```python
from build123d import *

# Parameters (mm, degrees)
BOSS_EXTRUDE2_DEPTH = 1000
CUT_EXTRUDE1_REACH  = 1002
SKETCH3_R           = 2
SKETCH3_R_2         = 1.999999992


with BuildPart() as part:
    # Sketch2 → Boss-Extrude2 (new body)
    with BuildSketch(Plane.XY):
        Polygon((0, 0), (0, 10), (0.7, 10), (0.7, 10.9), (2.2, 10.9), (2.2, 6.4), (4.9, 6.4), (9.142640687, 10.642640687), (9.142640687, 19.642640687), (4.9, 23.885281374), (2.2, 23.885281374), (2.2, 19.385281374), (0.7, 19.385281374), (0.7, 20.285281374), (0, 20.285281374), (0, 30.285281374), (10, 30.285281374), (10, 29.585281374), (10.9, 29.585281374), (10.9, 28.085281374), (6.4, 28.085281374), (6.4, 25.385281374), (10.642640687, 21.142640687), (19.642640687, 21.142640687), (23.885281374, 25.385281374), (23.885281374, 28.085281374), (19.385281374, 28.085281374), (19.385281374, 29.585281374), (20.285281374, 29.585281374), (20.285281374, 30.285281374), (30.285281374, 30.285281374), (30.285281374, 20.285281374), (29.585281374, 20.285281374), (29.585281374, 19.385281374), (28.085281374, 19.385281374), (28.085281374, 23.885281374), (25.385281374, 23.885281374), (21.142640687, 19.642640687), (21.142640687, 10.642640687), (25.385281374, 6.4), (28.085281374, 6.4), (28.085281374, 10.9), (29.585281374, 10.9), (29.585281374, 10), (30.285281374, 10), (30.285281374, 0), (20.285281374, 0), (20.285281374, 0.7), (19.385281374, 0.7), (19.385281374, 2.2), (23.885281374, 2.2), (23.885281374, 4.9), (19.642640687, 9.142640687), (10.642640687, 9.142640687), (6.4, 4.9), (6.4, 2.2), (10.9, 2.2), (10.9, 0.7), (10, 0.7), (10, 0), align=None)
    extrude(amount=-BOSS_EXTRUDE2_DEPTH)

    # Sketch3 → Cut-Extrude1 (cut, up to next)
    with BuildSketch(Plane.XY, mode=Mode.PRIVATE) as cut_extrude1_sk1:
        with Locations((3.200056686, 27.085348905)):
            Circle(SKETCH3_R)
    cut_extrude1_tool1 = extrude(cut_extrude1_sk1.sketch, amount=-CUT_EXTRUDE1_REACH, mode=Mode.PRIVATE) & part.part
    add(cut_extrude1_tool1.solids().sort_by_distance((3.200057, 27.085349, 0))[0], mode=Mode.SUBTRACT)
    # Sketch3 → Cut-Extrude1 (cut, up to next)
    with BuildSketch(Plane.XY, mode=Mode.PRIVATE) as cut_extrude1_sk2:
        with Locations((27.085224689, 27.085348905)):
            Circle(SKETCH3_R)
    cut_extrude1_tool2 = extrude(cut_extrude1_sk2.sketch, amount=-CUT_EXTRUDE1_REACH, mode=Mode.PRIVATE) & part.part
    add(cut_extrude1_tool2.solids().sort_by_distance((27.085225, 27.085349, 0))[0], mode=Mode.SUBTRACT)
    # Sketch3 → Cut-Extrude1 (cut, up to next)
    with BuildSketch(Plane.XY, mode=Mode.PRIVATE) as cut_extrude1_sk3:
        with Locations((27.085224689, 3.19993247)):
            Circle(SKETCH3_R)
    cut_extrude1_tool3 = extrude(cut_extrude1_sk3.sketch, amount=-CUT_EXTRUDE1_REACH, mode=Mode.PRIVATE) & part.part
    add(cut_extrude1_tool3.solids().sort_by_distance((27.085225, 3.199932, 0))[0], mode=Mode.SUBTRACT)
    # Sketch3 → Cut-Extrude1 (cut, up to next)
    with BuildSketch(Plane.XY, mode=Mode.PRIVATE) as cut_extrude1_sk4:
        with Locations((3.19993247, 3.200056686)):
            Circle(SKETCH3_R_2)
    cut_extrude1_tool4 = extrude(cut_extrude1_sk4.sketch, amount=-CUT_EXTRUDE1_REACH, mode=Mode.PRIVATE) & part.part
    add(cut_extrude1_tool4.solids().sort_by_distance((3.199932, 3.200057, 0))[0], mode=Mode.SUBTRACT)
    # Sketch3 → Cut-Extrude1 (cut, up to next)
    with BuildSketch(Plane.XY, mode=Mode.PRIVATE) as cut_extrude1_sk5:
        with BuildLine():
            Line((11.288922887, 17.865021836), (12.349577543, 16.804356148))
            ThreePointArc((12.349577543, 16.804356148), (11.892640687, 15.142640687), (12.349577543, 13.480925226))
            Line((12.349577543, 13.480925226), (11.288922887, 12.420259538))
            ThreePointArc((11.288922887, 12.420259538), (11.288928771, 11.288888688), (12.420299621, 11.288894572))
            Line((12.420299621, 11.288894572), (13.480954277, 12.34956026))
            ThreePointArc((13.480954277, 12.34956026), (15.142640687, 11.892640687), (16.804327097, 12.34956026))
            Line((16.804327097, 12.34956026), (17.864981753, 11.288894572))
            ThreePointArc((17.864981753, 11.288894572), (18.996352603, 11.288888688), (18.996358487, 12.420259538))
            Line((18.996358487, 12.420259538), (17.935703831, 13.480925226))
            ThreePointArc((17.935703831, 13.480925226), (18.392640687, 15.142640687), (17.935703831, 16.804356148))
            Line((17.935703831, 16.804356148), (18.996358487, 17.865021836))
            ThreePointArc((18.996358487, 17.865021836), (18.996352603, 18.996392686), (17.864981753, 18.996386802))
            Line((17.864981753, 18.996386802), (16.804327097, 17.935721114))
            ThreePointArc((16.804327097, 17.935721114), (15.142640687, 18.392640687), (13.480954277, 17.935721114))
            Line((13.480954277, 17.935721114), (12.420299621, 18.996386802))
            ThreePointArc((12.420299621, 18.996386802), (11.288928771, 18.996392686), (11.288922887, 17.865021836))
        make_face()
    cut_extrude1_tool5 = extrude(cut_extrude1_sk5.sketch, amount=-CUT_EXTRUDE1_REACH, mode=Mode.PRIVATE) & part.part
    add(cut_extrude1_tool5.solids().sort_by_distance((15.142641, 15.142641, 0))[0], mode=Mode.SUBTRACT)


solid = part.part
```
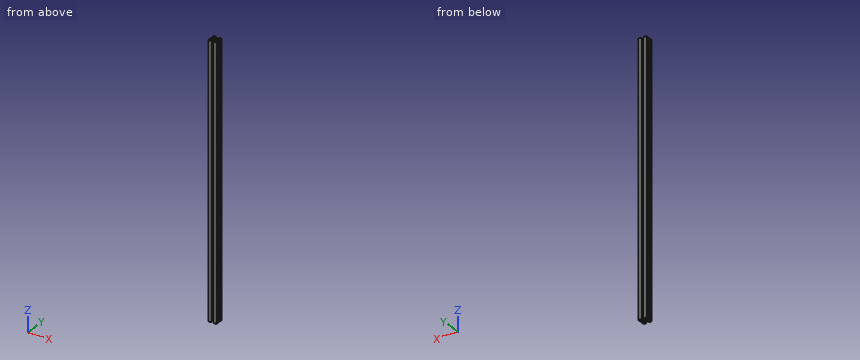
Work out the finished part from the listing and answer in its coordinate system (mm). Give positions to 0.01 mm unless a question says otherwise; leave off trailing zeros. Put each result on its own line as item: value. Start each with the question number.
Item 1: Find the intervals of material crossed by L1, parallel to Y at x = 18, z = -128; L2, parallel to X at y = 27, z = -764.5; L3, parallel to Y at x = 3, z = -494.5, in increasing order. Write a range as [from, to].
Item 2: Each of these flat-tipped pins is pushed along its axis until it touches: P1, Ø1, axis at x = 17, z = -231, coming from the -Y side; P2, Ø6, axis at y = 16, z = -419.5, coming from the +X side; P3, Ø3, axis at y = 15.5, z = -561.5, coming from the -X side. Where does it stop, or does it pass through?
Item 3: The part is cut by section A-A (z = -521.5). State how many separate pieces and enclosed holes the cut face has, then the cut area to 3 significant figures.
Answers below:
1. L1: [9.14, 11.18], [13.42, 13.59], [16.69, 16.87], [19.1, 21.14]
1. L2: [0, 1.2], [5.2, 6.4], [23.89, 25.09], [29.08, 30.29]
1. L3: [0, 1.21], [5.19, 6.4], [23.89, 25.1], [29.08, 30.29]
2. P1: y = 9.14
2. P2: x = 21.14
2. P3: x = 9.14
3. separate pieces: 1
3. enclosed holes: 5
3. area: 327 mm2
